Could you check a few things on this model? Use its own coordinates, in mm. A direction names the side the tool comes from. Coordinates: 2 decimals unless noted, no trailing zeros. Write each loop counter-clockwise with the first axis right and the second up, starting at its lowest first coordinate (ties: lowest second). Pieces come first, ordered by that corner, then holes. Notation, with made-up numbers: (82.25, 81) - (102.25, 81) arc R26 ccw to (102.25, 118) - close; hole circle Ø7 at (77, 64). An arc over 180 degrees is marked (long way). Answer as a JSON object with one key per item and string values. Group by question number.
1) If we section it at B-B (y = 0): Write out the boundary of the cut face in (x, z), plus the area to 3 significant figures.
2) On a 3-axis mill with a long thin cutter (end or side, diameter ignored), from which of +Z, -Z, +X, -X, +Y, -Y can I reach the whole of each face in a straight line? I mean faces 4 (the cylindrical face through (10.398, 0.106, -0.838)), 5 (the flat face through (-3.9, 0, 8)), 6 (the flat face through (11.9, 0, 5)). Say none if no direction works.
3) If we section it at C-C (x = 8): Write out the boundary of the cut face in (y, z), plus the area to 3 significant figures.
4) If we section it at A-A (z = 5): Write out the boundary of the cut face in (x, y).
5) Will this pin go through, and if not, where does the flat tip stop? pin 1 Ø1 at (x, y) = (0, 2) entering from +Z.
6) Please list where these lines run through material, in increasing order: line 1 along X through (y, z) = (-0.5, 7.75); line 2 along Z through (x, y) = (8, -3); line 3 along X through (y, z) = (2.5, 4.75).
7) If we section it at D-D (y = 2.75): Write out the boundary of the cut face in (x, z).
8) We'd pull the mould along X, two halves only. Please class faces 1 (the flat face through (-11.9, 0, 5)), 2 (the flat face through (0, 0, -1.7)), 3 (the flat face through (3.9, 0, 8)): released by +X, released by -X, zero draft, split by the parting line, or undercut.
```python
from build123d import *

# Parameters (mm, degrees)
SKETCH_1_W          = 23.8
SKETCH_1_H          = 7.8
EXTRUDE_1_DEPTH     = 9.6
SKETCH_2_R          = 2.4
EXTRUDE_2_DEPTH     = 1.7
CUT_EXTRUDE_1_DEPTH = 18.164206944


with BuildPart() as part:
    # Эскиз1 → Бобышка-Вытянуть1 (new body)
    with BuildSketch(Plane.XY):
        Rectangle(SKETCH_1_W, SKETCH_1_H)
    extrude(amount=EXTRUDE_1_DEPTH)

    # Эскиз2 → Бобышка-Вытянуть2 (add)
    with BuildSketch(Plane(origin=(0, 0, 0), x_dir=(-1, 0, 0), z_dir=(0, 0, -1))):
        Circle(SKETCH_2_R)
        with Locations((8, 0)):
            Circle(SKETCH_2_R)
        with Locations((-8, 0)):
            Circle(SKETCH_2_R)
    extrude(amount=EXTRUDE_2_DEPTH)

    # Эскиз3 → Вырез-Вытянуть1 (cut, through all)
    with BuildSketch(Plane(origin=(0, 3.9, 0), x_dir=(1, 0, 0), z_dir=(0, 1, 0))):
        with BuildLine():
            Line((-3.9, -16.6), (3.9, -16.6))
            Line((3.9, -16.6), (3.9, -6.5))
            ThreePointArc((3.9, -6.5), (0, -2.6), (-3.9, -6.5))
            Line((-3.9, -6.5), (-3.9, -16.6))
        make_face()
    extrude(amount=-CUT_EXTRUDE_1_DEPTH, mode=Mode.SUBTRACT)


solid = part.part
```
Here are the results:
{
 "1": {"outline": "(-11.9, 0) - (-10.4, 0) - (-10.4, -1.7) - (-5.6, -1.7) - (-5.6, 0) - (-2.4, 0) - (-2.4, -1.7) - (2.4, -1.7) - (2.4, 0) - (5.6, 0) - (5.6, -1.7) - (10.4, -1.7) - (10.4, 0) - (11.9, 0) - (11.9, 9.6) - (3.9, 9.6) - (3.9, 6.5) arc R3.9 cw to (-3.9, 6.5) - (-3.9, 9.6) - (-11.9, 9.6) - close", "area": "205 mm²"},
 "2": {"face 4": "-Z", "face 5": "+Z, +Y, -Y", "face 6": "+Z, -Z, +X, +Y, -Y"},
 "3": {"outline": "(-3.9, 0) - (-2.4, 0) - (-2.4, -1.7) - (2.4, -1.7) - (2.4, 0) - (3.9, 0) - (3.9, 9.6) - (-3.9, 9.6) - close", "area": "83.0 mm²"},
 "4": {"outline": "(-11.9, -3.9) - (-3.6, -3.9) - (-3.6, 3.9) - (-11.9, 3.9) - close; (3.6, -3.9) - (11.9, -3.9) - (11.9, 3.9) - (3.6, 3.9) - close"},
 "5": {"pin 1": "stops at z = 2.63"},
 "6": {"line 1": "x = -11.9 to -3.9, 3.9 to 11.9", "line 2": "z = 0 to 9.6", "line 3": "x = -11.9 to -3.49, 3.49 to 11.9"},
 "7": {"outline": "(-11.9, 0) - (11.9, 0) - (11.9, 9.6) - (3.9, 9.6) - (3.9, 6.5) arc R3.9 cw to (-3.9, 6.5) - (-3.9, 9.6) - (-11.9, 9.6) - close"},
 "8": {"face 1": "released by -X", "face 2": "zero draft", "face 3": "undercut"}
}
